from build123d import *

# Parameters (mm, degrees)
F0_W           = 35.56
F0_H           = 67.31
F0_W_2         = 31.75
F0_H_2         = 31.75
F1_DEPTH       = 2.54
F3_D           = 3.175
F3_CSINK_D     = 6.858
F3_CSINK_ANGLE = 90
F4_D           = 3.175
F6_DEPTH       = 3.175
F7_DEPTH       = 4.699


with BuildPart() as f1:
    # F0 (on Top) → F1 (new body)
    with BuildSketch(Plane.XY):
        Rectangle(F0_W, F0_H)
        Rectangle(F0_W_2, F0_H_2, mode=Mode.SUBTRACT)
    extrude(amount=F1_DEPTH)

    # F3 (through all)
    with Locations(Plane.XY.offset(2.54)):
        with Locations((0, 29.21), (0, -29.21)):
            CounterSinkHole(F3_D / 2, F3_CSINK_D / 2, counter_sink_angle=F3_CSINK_ANGLE)

    # F4 (through all)
    with Locations(Plane(origin=(0, 0, 0), x_dir=(1, 0, 0), z_dir=(0, 0, -1))):
        with Locations((0, -18.542), (0, 18.542)):
            Hole(F4_D / 2)

    # F5 (on face) → F6 (join)
    with BuildSketch(Plane.XY.offset(2.54)):
        Polygon((-15.24, 33.655), (-16.51, 33.655), (-16.51, -33.655), (-15.24, -33.655), (-15.24, -15.875), (-15.875, -15.875), (-15.875, 15.875), (-15.24, 15.875), align=None)
        Polygon((16.51, 33.655), (15.24, 33.655), (15.24, 15.875), (15.875, 15.875), (15.875, -15.875), (15.24, -15.875), (15.24, -33.655), (16.51, -33.655), align=None)
    extrude(amount=F6_DEPTH)

    # F7 (add): faces of the model
    f7_faces = [f1.faces().sort_by_distance(p)[0] for p in [
        (-17.145, 0, 2.54),
        (17.145, 0, 2.54),
    ]]
    extrude(f7_faces, amount=F7_DEPTH)


solid = f1.part
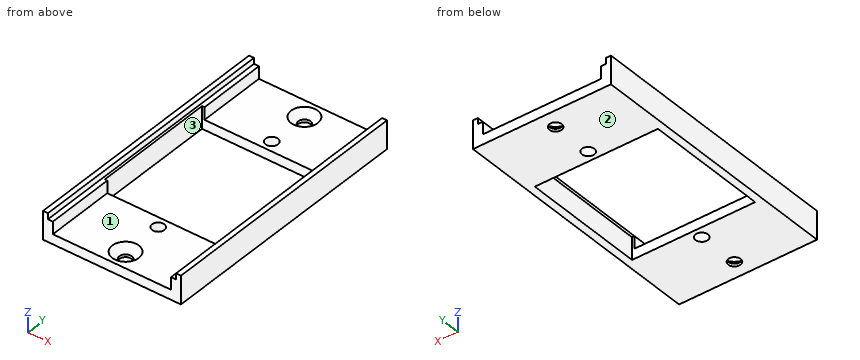
Can you work these out from the model? Positions are in its coordinate system, mm. Face numbers are marked on the shaded views. A direction names the side the tool comes from. Round coordinates to 2 decimals unless told otherwise and drop trailing zeros. Order: outer loops, then holes, each group sorted by start corner. A loop starts at its lowest first (then second) coordinate and runs counter-clockwise, first axis right, second up. Notation, with made-up numbers: (-17, 12.5) -> (21, 12.5) arc R37 cw to (21, 51.5) -> close; hole circle Ø6 at (-14, 24). An arc over 180 degrees is marked (long way). Write each question's results on one line, items separated by ' | '. Start each with the question number.
Item 1: If we section it at A-A, the plane x = 0: Write out the boundary of the cut face in (y, z) (1 decimal).
Item 2: If we section it at C-C, the plane z = 4.25: Write out the boundary of the cut face in (x, y) (3 decimals), then the cut area to 3 significant figures.
Item 3: Which directions (+Z, -Z, +X, -X, +Y, -Y) give clear straight access to the entire face, cutting with the end or side of a thin tool? Please do the marked faces 1, 2 and 3.
Item 4: If we section it at D-D, the plane x = -10: Write out the boundary of the cut face in (y, z) (3 decimals).
Item 5: If we section it at B-B, the plane y = -29.21: Write out the boundary of the cut face in (x, z) (1 decimal), then the cut area to 3 significant figures.
Item 6: Please list where these lines run through material, in increasing order: L1, parallel to Y at x = 0, z = 0.3 (1 decimal); L2, parallel to X at y = 9, z = 1.75 (3 decimals); L3, parallel to Y at x = -11, z = 1.25 (3 decimals).
Results:
1) outline: (-33.7, 0) -> (-30.8, 0) -> (-30.8, 0.7) -> (-32.6, 2.5) -> (-33.7, 2.5) -> close; (-27.6, 0) -> (-20.1, 0) -> (-20.1, 2.5) -> (-25.8, 2.5) -> (-27.6, 0.7) -> close; (-17, 0) -> (-15.9, 0) -> (-15.9, 2.5) -> (-17, 2.5) -> close; (15.9, 0) -> (17, 0) -> (17, 2.5) -> (15.9, 2.5) -> close; (20.1, 0) -> (27.6, 0) -> (27.6, 0.7) -> (25.8, 2.5) -> (20.1, 2.5) -> close; (30.8, 0) -> (33.7, 0) -> (33.7, 2.5) -> (32.6, 2.5) -> (30.8, 0.7) -> close
2) outline: (-17.78, -33.655) -> (-15.24, -33.655) -> (-15.24, -15.875) -> (-15.875, -15.875) -> (-15.875, 15.875) -> (-15.24, 15.875) -> (-15.24, 33.655) -> (-17.78, 33.655) -> close; (15.24, -33.655) -> (17.78, -33.655) -> (17.78, 33.655) -> (15.24, 33.655) -> (15.24, 15.875) -> (15.875, 15.875) -> (15.875, -15.875) -> (15.24, -15.875) -> close | area: 302 mm2
3) face 1: +Z, +Y, -Y | face 2: -Z, +X, -X, +Y, -Y | face 3: +Z, -Z
4) outline: (-33.655, 0) -> (-15.875, 0) -> (-15.875, 2.54) -> (-33.655, 2.54) -> close; (15.875, 0) -> (33.655, 0) -> (33.655, 2.54) -> (15.875, 2.54) -> close
5) outline: (-17.8, 0) -> (-1.6, 0) -> (-1.6, 0.7) -> (-3.4, 2.5) -> (-15.2, 2.5) -> (-15.2, 5.7) -> (-16.5, 5.7) -> (-16.5, 7.2) -> (-17.8, 7.2) -> close; (1.6, 0) -> (17.8, 0) -> (17.8, 7.2) -> (16.5, 7.2) -> (16.5, 5.7) -> (15.2, 5.7) -> (15.2, 2.5) -> (3.4, 2.5) -> (1.6, 0.7) -> close | area: 98.9 mm2
6) L1: y = -33.7 to -30.8, -27.6 to -20.1, -17 to -15.9, 15.9 to 17, 20.1 to 27.6, 30.8 to 33.7 | L2: x = -17.78 to -15.875, 15.875 to 17.78 | L3: y = -33.655 to -15.875, 15.875 to 33.655
